Check sheet for the modelled part. Datum: model origin and axes. Units: mm. Face numbers are marked on the shaded views. A direction names the side the tool comes from. Round coordinates to 2 decimals unless told otherwise and drop trailing zeros. Order: outer loops, then holes, each group sorted by start corner. A loop starts at its lowest first (then second) coordinate and runs counter-clockwise, first axis right, second up. Notation, with made-up numbers: M -29,-33.75 L -15,-33.75 A10 cw -15,-14.75 Z; hole C 67,-6 d4. An arc over 180 degrees is marked long. One line per item, written item: value. Start each with the question number.
(1) Cross-section at B-B, the plane z = 5.25. Enter the section's corners in (x, y).
(2) Thickness scan on L1, parallel to Y at x = 7.5, z = 0; L2, parallel to X at y = 4, z = 10.25; L3, parallel to Y at x = 27.2, z = 0. Record the ranges inside material, lowest first.
(3) Access from +Z, -Z, +X, -X, +Y, -Y to the whole of each face (thin tool, end or side, straight path). Record for the marked faces 4, 5 and 6.
(4) Cross-section at D-D, the plane z = -8.5. Enter the section's corners in (x, y).
(5) Depth check by flat-ended pin: pin 1 Ø5 at (y, z) = (0.5, -0.5) entering from -X; pin 2 Ø6 at (y, z) = (-0.5, -2.5) entering from -X; pin 3 Ø2 at (x, y) = (57, -8.5) entering from -Z. Enter the tip coordinate at first touch or a pass-through.
(6) Release check for a two-part mould opening along Z. For the marked faces 1, 2 and 3 record: released by +Z, released by -Z, zero draft, split by the parting line, or undercut.
(7) Cross-section at A-A, the plane x = 15. Enter the section's corners in (y, z).
(8) Cross-section at C-C, the plane x = 42. Enter the section's corners in (y, z), and give its area (3 significant figures).
from build123d import *

# Parameters (mm, degrees)
SKIZZE1_R                       = 11.5
AUFSATZ_LINEAR_AUSTRAGEN1_DEPTH = 77
SKIZZE2_R                       = 7.1
SCHNITT_LINEAR_AUSTRAGEN1_DEPTH = 4.1
SKIZZE3_R                       = 4.25
SCHNITT_LINEAR_AUSTRAGEN2_DEPTH = 43
SKIZZE4_R                       = 9.6
SCHNITT_LINEAR_AUSTRAGEN3_DEPTH = 12.75
SCHNITT_LINEAR_START            = -6
SKIZZE7_W                       = 1.5
SKIZZE7_H                       = 15
SCHNITT_LINEAR_AUSTRAGEN4_DEPTH = 63
SKIZZE8_W                       = 63
SKIZZE8_H                       = 4
AUFSATZ_LINEAR_AUSTRAGEN2_DEPTH = 1.5
SCHNITT_LINEAR_AUSTRAGEN6_DEPTH = 13.5
SKIZZE12_R                      = 3
SCHNITT_LINEAR_AUSTRAGEN7_DEPTH = 2
KREISMUSTER3_COUNT              = 3


with BuildPart() as part:
    # Skizze1 → Aufsatz-Linear austragen1 (new body)
    with BuildSketch(Plane(origin=(0, 0, 0), x_dir=(0, 0, -1), z_dir=(1, 0, 0))):
        Circle(SKIZZE1_R)
    extrude(amount=AUFSATZ_LINEAR_AUSTRAGEN1_DEPTH)

    # Skizze2 → Schnitt-Linear austragen1 (cut)
    with BuildSketch(Plane(origin=(77, 0, 0), x_dir=(0, 0, -1), z_dir=(1, 0, 0))):
        Circle(SKIZZE2_R)
    extrude(amount=-SCHNITT_LINEAR_AUSTRAGEN1_DEPTH, mode=Mode.SUBTRACT)

    # Skizze3 → Schnitt-Linear austragen2 (cut)
    with BuildSketch(Plane(origin=(72.9, 0, 0), x_dir=(0, 0, -1), z_dir=(1, 0, 0))):
        Circle(SKIZZE3_R)
    extrude(amount=-SCHNITT_LINEAR_AUSTRAGEN2_DEPTH, mode=Mode.SUBTRACT)

    # Skizze4 → Schnitt-Linear austragen3 (cut)
    with BuildSketch(Plane.ZY):
        Circle(SKIZZE4_R)
    extrude(amount=-SCHNITT_LINEAR_AUSTRAGEN3_DEPTH, mode=Mode.SUBTRACT)

    # Skizze7 → Schnitt-Linear austragen4 (cut)
    with BuildSketch(Plane(origin=(77, 0, 0), x_dir=(0, 0, -1), z_dir=(1, 0, 0)).offset(SCHNITT_LINEAR_START)):
        with Locations((-10.75, 0)):
            Rectangle(SKIZZE7_W, SKIZZE7_H)
    schnitt_linear_austragen4 = extrude(amount=-SCHNITT_LINEAR_AUSTRAGEN4_DEPTH, mode=Mode.SUBTRACT)

    # Skizze8 → Aufsatz-Linear austragen2 (add)
    with BuildSketch(Plane.XY.offset(10)):
        with Locations((39.5, 0)):
            Rectangle(SKIZZE8_W, SKIZZE8_H)
    aufsatz_linear_austragen2 = extrude(amount=AUFSATZ_LINEAR_AUSTRAGEN2_DEPTH)

    # Skizze10 → Schnitt-Linear austragen6 (cut)
    with BuildSketch(Plane.ZY.offset(-12.75)):
        Polygon((4.038863706, -2.240739453), (3.959969143, 2.377388845), (-0.078894563, 4.618128298), (-4.038863706, 2.240739453), (-3.959969143, -2.377388845), (0.078894563, -4.618128298), align=None)
    extrude(amount=-SCHNITT_LINEAR_AUSTRAGEN6_DEPTH, mode=Mode.SUBTRACT)

    # Skizze12 → Schnitt-Linear austragen7 (cut)
    with BuildSketch(Plane.ZY.offset(-26.25)):
        Circle(SKIZZE12_R)
    extrude(amount=-SCHNITT_LINEAR_AUSTRAGEN7_DEPTH, mode=Mode.SUBTRACT)

    # Kreismuster3: Schnitt-Linear austragen4, Aufsatz-Linear austragen2 ×3 about axis
    kreismuster3_axis = Axis((0, 0, 0), (1, 0, 0))
    add([schnitt_linear_austragen4.rotate(kreismuster3_axis, i * 360 / KREISMUSTER3_COUNT) for i in range(1, KREISMUSTER3_COUNT)], mode=Mode.SUBTRACT)
    add([aufsatz_linear_austragen2.rotate(kreismuster3_axis, i * 360 / KREISMUSTER3_COUNT) for i in range(1, KREISMUSTER3_COUNT)])


solid = part.part
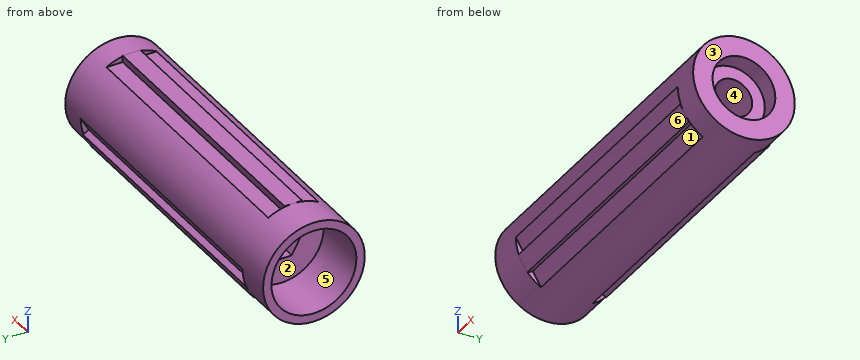
Values found:
1. outline: M 0,-10.23 L 77,-10.23 L 77,-4.78 L 72.9,-4.78 L 72.9,4.78 L 77,4.78 L 77,10.23 L 0,10.23 L 0,8.04 L 12.75,8.04 L 12.75,-8.04 L 0,-8.04 Z
2. L1: -11.5 to -9.6, 9.6 to 11.5
2. L2: 0 to 8, 71 to 77
2. L3: -11.5 to -3, 3 to 11.5
3. face 4: +X
3. face 5: -X
3. face 6: -Z, +X, -X, -Y
4. outline: M 0,-7.75 L 8,-7.75 L 8,-6.64 L 71,-6.64 L 71,-7.75 L 77,-7.75 L 77,7.75 L 71,7.75 L 71,6.64 L 8,6.64 L 8,7.75 L 0,7.75 L 0,4.46 L 12.75,4.46 L 12.75,-4.46 L 0,-4.46 Z
5. pin 1: x = 26.25
5. pin 2: x = 12.75
5. pin 3: z = -7.48
6. face 1: released by -Z
6. face 2: undercut
6. face 3: zero draft
7. outline: M -11.5,-0.08 L -9.66,-3.27 L -10.96,-4.02 L -8.96,-7.48 L -7.66,-6.73 L -5.82,-9.92 A11.5 ccw 5.82,-9.92 L 7.66,-6.73 L 8.96,-7.48 L 10.96,-4.02 L 9.66,-3.27 L 11.5,-0.08 A11.5 ccw 5.68,10 L 2,10 L 2,11.5 L -2,11.5 L -2,10 L -5.68,10 A11.5 ccw Z; hole M -4.62,0.08 L -2.38,-3.96 L 2.24,-4.04 L 4.62,-0.08 L 2.38,3.96 L -2.24,4.04 Z
8. outline: M -11.5,-0.08 L -9.66,-3.27 L -10.96,-4.02 L -8.96,-7.48 L -7.66,-6.73 L -5.82,-9.92 A11.5 ccw 5.82,-9.92 L 7.66,-6.73 L 8.96,-7.48 L 10.96,-4.02 L 9.66,-3.27 L 11.5,-0.08 A11.5 ccw 5.68,10 L 2,10 L 2,11.5 L -2,11.5 L -2,10 L -5.68,10 A11.5 ccw Z; hole C 0,0 d8.5
8. area: 342 mm^2
